Source: three-view drawing plus pictorial views. Frame: mm from the lowest corner of the part. Round coordinates to 2 decimals unless told otherwise and drop trailing zeros. Order: outer loops, then holes, each group sorted by start corner. A loop starts at its lowest first (then second) coordinate and runs counter-clockwise, first axis right, second up. Notation, with made-up numbers: (77.5, -37) -> (81.5, -37) arc R22 ccw to (81.5, -17) -> close; hole circle Ø6 at (-20.75, 65.25). An arc over 180 degrees is marked (long way). Answer as CSV lines item,"result".
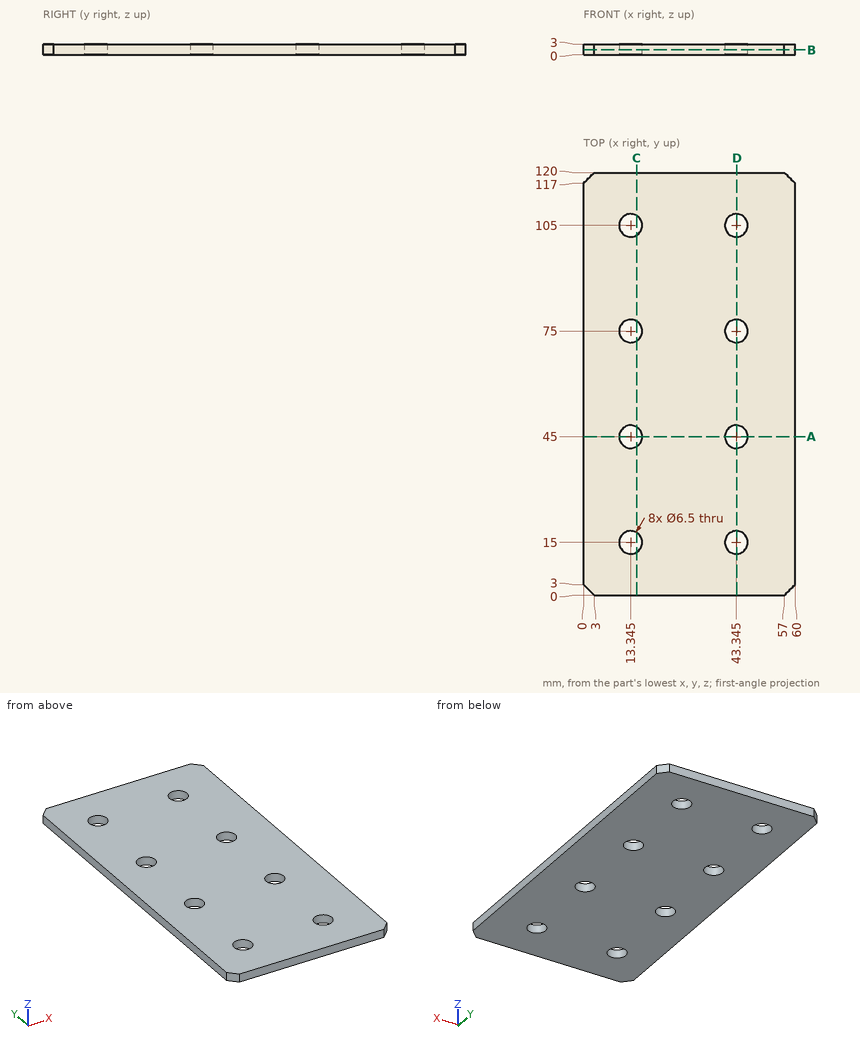
1. Section query D-D on x = 43.5. Return loops of the section in (y, z), and give its area (3 significant figures).
Results below:
outline,"(0, 0) -> (11.75, 0) -> (11.75, 3) -> (0, 3) -> close; (18.25, 0) -> (41.75, 0) -> (41.75, 3) -> (18.25, 3) -> close; (48.25, 0) -> (71.75, 0) -> (71.75, 3) -> (48.25, 3) -> close; (78.25, 0) -> (101.75, 0) -> (101.75, 3) -> (78.25, 3) -> close; (108.25, 0) -> (120, 0) -> (120, 3) -> (108.25, 3) -> close"
area,"282 mm2"
2. Line query: L1, parallel to X at y = 17, z = 2.1; L2, parallel to Y at x = 44, z = 0.6; L3, parallel to X at y = 44, z = 0.7. Output: solid intervals per line, ascending. Write a range as [from, to].
Results below:
L1,"[0, 10.78], [15.91, 40.78], [45.91, 60]"
L2,"[0, 11.82], [18.18, 41.82], [48.18, 71.82], [78.18, 101.82], [108.18, 120]"
L3,"[0, 10.25], [16.44, 40.25], [46.44, 60]"
3. Section query B-B on z = 1.3. Give the number of separate pieces and of enclosed holes in the cut face, and give its area (3 significant figures).
Results below:
separate pieces,"1"
enclosed holes,"8"
area,"6,920 mm2"
4. Section query A-A on y = 45. Return loops of the section in (x, z) (3 decimals).
Results below:
outline,"(0, 0) -> (10.095, 0) -> (10.095, 3) -> (0, 3) -> close; (16.595, 0) -> (40.095, 0) -> (40.095, 3) -> (16.595, 3) -> close; (46.595, 0) -> (60, 0) -> (60, 3) -> (46.595, 3) -> close"
5. Section query C-C on x = 15. Return loops of the section in (y, z), and give its area (3 significant figures).
Results below:
outline,"(0, 0) -> (12.2, 0) -> (12.2, 3) -> (0, 3) -> close; (17.8, 0) -> (42.2, 0) -> (42.2, 3) -> (17.8, 3) -> close; (47.8, 0) -> (72.2, 0) -> (72.2, 3) -> (47.8, 3) -> close; (77.8, 0) -> (102.2, 0) -> (102.2, 3) -> (77.8, 3) -> close; (107.8, 0) -> (120, 0) -> (120, 3) -> (107.8, 3) -> close"
area,"293 mm2"
6. Pin query (flat end, axial travel): pin 1 (4 mm diameter, centred on x = 13.35, y = 45, fed in from -Z). Return the tip coordinate at first contact, or that it passes through.
Results below:
pin 1,"through"
